Build history of the part. All positions in model axes, mm. A direction names the side the tool comes from. Give positions to 0.01 mm unless a question says otherwise; leave off trailing zeros. Order: outer loops, then holes, each group sorted by start corner. A loop starts at its lowest first (then second) coordinate and runs counter-clockwise, first axis right, second up. Notation, with made-up numbers: (1.5, 56.5) - (13.5, 56.5) arc R25 ccw to (13.5, 69.5) - close; hole circle Ø5 at (-7, -14). An arc over 180 degrees is marked (long way). Use a Markdown table: item, result. Add a question column.
(1) Which spindle directions (+Z, -Z, +X, -X, +Y, -Y) get a long thin tool onto all of the face, cutting with end or side? Do faces 1 (the face through (-1.23, 15.61, 5)), 2 (the face through (-2.75, 11, 11)), 3 (the face through (0.25, -8, 11)). Say none if no direction does.
(2) Slice it at A-A (y = -18). Write the cut outline in (x, z), then the cut area to 3 significant figures.
(3) Mould opens along Y. For faces 4 (the face through (-20, -19.8, 11)), 5 (the face through (-38.729, 10.271, 11.315)), 6 (the face through (97.25, -21, 21)) say: +Y half, -Y half, draft (parallel to the pull), parting line (faces both ways), or undercut.
(4) Flat gauge pins, fed straight in: pin 1 (2 mm diameter, centred on x = -17, y = -20.5, fed in from -Z); pin 2 (3 mm diameter, centred on y = 9.85, z = 29.65, fed in from +X); pin 3 (1.5 mm diameter, centred on x = -10, z = 6, fed in from +Y). Where does each tip first touch, or does it go through?
(5) Slice it at D-D (y = 16.85). Write the cut outline in (x, z), then the cut area to 3 significant figures.
(6) Slice it at C-C (z = 21.15). Write the cut outline in (x, y), then the cut area to 3 significant figures.
(7) Slice it at B-B (x = -10.5). Write the cut outline in (y, z).
(8) Wall check: line 1 (Z direction, x = -1, y = -14); line 2 (Y direction, x = -38.45, z = 29.65); line 3 (X direction, y = 2, z = 4). Give the ranges that are in metal, low to high.
from build123d import *

# Parameters (mm, degrees)
BOSS_EXTRUDE1_DEPTH = 42.3
SKETCH3_R           = 11.5
SKETCH3_R_2         = 1.4
CUT_EXTRUDE1_DEPTH  = 5
SKETCH4_R           = 1.4
CUT_EXTRUDE2_DEPTH  = 5
SKETCH5_W           = 20
SKETCH5_H           = 10
CUT_EXTRUDE3_DEPTH  = 5


with BuildPart() as part:
    # Sketch2 → Boss-Extrude1 (new body)
    with BuildSketch(Plane.XY):
        Polygon((-2.75, 22.5), (-2.75, -19.8), (-37.25, -19.8), (-37.25, 22.5), (-40.25, 22.5), (-40.25, -22.5), (97.25, -22.5), (97.25, -19.8), (0.25, -19.8), (0.25, 22.5), align=None)
    extrude(amount=BOSS_EXTRUDE1_DEPTH)

    # Sketch3 → Cut-Extrude1 (cut)
    with BuildSketch(Plane(origin=(0.25, 0, 0), x_dir=(0, 0, -1), z_dir=(1, 0, 0))):
        with Locations((-21.15, 1.35)):
            Circle(SKETCH3_R)
        with Locations((-36.65, 16.85)):
            Circle(SKETCH3_R_2)
        with Locations((-5.65, 16.85)):
            Circle(SKETCH3_R_2)
        with Locations((-5.65, -14.15)):
            Circle(SKETCH3_R_2)
        with Locations((-36.65, -14.15)):
            Circle(SKETCH3_R_2)
    extrude(amount=-CUT_EXTRUDE1_DEPTH, mode=Mode.SUBTRACT)

    # Sketch4 → Cut-Extrude2 (cut)
    with BuildSketch(Plane(origin=(-37.25, 0, 0), x_dir=(0, 0, -1), z_dir=(1, 0, 0))):
        with Locations((-29.65, 9.85)):
            Circle(SKETCH4_R)
        with Locations((-12.65, 9.85)):
            Circle(SKETCH4_R)
        with Locations((-12.65, -7.15)):
            Circle(SKETCH4_R)
        with Locations((-29.65, -7.15)):
            Circle(SKETCH4_R)
    extrude(amount=-CUT_EXTRUDE2_DEPTH, mode=Mode.SUBTRACT)

    # Sketch5 → Cut-Extrude3 (cut)
    with BuildSketch(Plane(origin=(0, -19.8, 0), x_dir=(1, 0, 0), z_dir=(0, 1, 0))):
        with Locations((-19.25, -21.070122094)):
            Rectangle(SKETCH5_W, SKETCH5_H)
    extrude(amount=-CUT_EXTRUDE3_DEPTH, mode=Mode.SUBTRACT)


solid = part.part
Solution:
| question | item | result |
|---|---|---|
| 1 | face 1 | +X |
| 1 | face 2 | +Z, -Z, +Y |
| 1 | face 3 | +Z, -Z, +X, +Y |
| 2 | outline | (-40.25, 0) - (-37.25, 0) - (-37.25, 42.3) - (-40.25, 42.3) - close; (-2.75, 0) - (0.25, 0) - (0.25, 42.3) - (-2.75, 42.3) - close |
| 2 | area | 254 mm2 |
| 3 | face 4 | +Y half |
| 3 | face 5 | undercut |
| 3 | face 6 | draft |
| 4 | pin 1 | z = 0 |
| 4 | pin 2 | x = 0.25 |
| 4 | pin 3 | y = -19.8 |
| 5 | outline | (-40.25, 0) - (-37.25, 0) - (-37.25, 42.3) - (-40.25, 42.3) - close; (-2.75, 0) - (0.25, 0) - (0.25, 4.25) - (-2.75, 4.25) - close; (-2.75, 7.05) - (0.25, 7.05) - (0.25, 35.25) - (-2.75, 35.25) - close; (-2.75, 38.05) - (0.25, 38.05) - (0.25, 42.3) - (-2.75, 42.3) - close |
| 5 | area | 237 mm2 |
| 6 | outline | (-40.25, -22.5) - (-29.25, -22.5) - (-29.25, -19.8) - (-37.25, -19.8) - (-37.25, 22.5) - (-40.25, 22.5) - close; (-9.25, -22.5) - (97.25, -22.5) - (97.25, -19.8) - (0.25, -19.8) - (0.25, -10.15) - (-2.75, -10.15) - (-2.75, -19.8) - (-9.25, -19.8) - close; (-2.75, 12.85) - (0.25, 12.85) - (0.25, 22.5) - (-2.75, 22.5) - close |
| 6 | area | 502 mm2 |
| 7 | outline | (-22.5, 0) - (-19.8, 0) - (-19.8, 16.07) - (-22.5, 16.07) - close; (-22.5, 26.07) - (-19.8, 26.07) - (-19.8, 42.3) - (-22.5, 42.3) - close |
| 8 | line 1 | 0 to 4.26, 7.04 to 35.26, 38.04 to 42.3 |
| 8 | line 2 | -22.5 to -8.55, -5.75 to 8.45, 11.25 to 22.5 |
| 8 | line 3 | -40.25 to -37.25, -2.75 to 0.25 |
